Geometry check sheet. Reference: the model listing, model coordinates, mm. A direction names the side the tool comes from. Round coordinates to 2 decimals unless told otherwise and drop trailing zeros. Write each loop counter-clockwise with the first axis right and the second up, starting at its lowest first coordinate (ties: lowest second). Pieces come first, ordered by that corner, then holes. Notation, with made-up numbers: (40, 19) -> (69, 19) arc R8 ccw to (69, 31) -> close; hole circle Ø2 at (22.5, 48). An arc over 180 degrees is marked (long way). One line per question, with ' | ' between items.
```python
from build123d import *

# Parameters (mm, degrees)
ESQUISSE1_R             = 2.5
EXTRUSION1_DEPTH        = 14
ENL_V_MAT_EXTRU_1_DEPTH = 4
ESQUISSE4_R             = 2.5
ENL_V_MAT_EXTRU_2_DEPTH = 3
CHANFREIN1_SIZE         = 1


with BuildPart() as part:
    # Esquisse1 → Extrusion1 (new body)
    with BuildSketch(Plane.XY):
        with BuildLine():
            Line((-1.673913043, 5.239085333), (-12.108695652, 1.905121939))
            ThreePointArc((-12.108695652, 1.905121939), (-13.5, 0), (-12.108695652, -1.905121939))
            Line((-12.108695652, -1.905121939), (-1.673913043, -5.239085333))
            ThreePointArc((-1.673913043, -5.239085333), (5.5, 0), (-1.673913043, 5.239085333))
        make_face()
        Circle(ESQUISSE1_R, mode=Mode.SUBTRACT)
    extrude(amount=EXTRUSION1_DEPTH)

    # Esquisse2 → Enlèv. mat.-Extru.1 (cut)
    with BuildSketch(Plane.XY.offset(14)):
        with BuildLine():
            Line((-1.673913043, 5.239085333), (-7.389278861, 3.412998376))
            Line((-7.389278861, 3.412998376), (-6.298809411, 0))
            Line((-6.298809411, 0), (-7.389278861, -3.412998376))
            Line((-7.389278861, -3.412998376), (-1.673913043, -5.239085333))
            ThreePointArc((-1.673913043, -5.239085333), (5.5, 0), (-1.673913043, 5.239085333))
        make_face()
    extrude(amount=-ENL_V_MAT_EXTRU_1_DEPTH, mode=Mode.SUBTRACT)

    # Esquisse4 → Enlèv. mat.-Extru.2 (cut)
    with BuildSketch(Plane(origin=(0, 0, 0), x_dir=(-1, 0, 0), z_dir=(0, 0, -1))):
        Circle(ESQUISSE4_R)
        with BuildLine():
            Line((1.673913043, -5.239085333), (12.108695652, -1.905121939))
            ThreePointArc((12.108695652, -1.905121939), (13.5, 0), (12.108695652, 1.905121939))
            Line((12.108695652, 1.905121939), (1.673913043, 5.239085333))
            ThreePointArc((1.673913043, 5.239085333), (0.847062769, 5.434379879), (0, 5.5))
            Line((0, 5.5), (-1.881110788, -5.168309414))
            ThreePointArc((-1.881110788, -5.168309414), (-0.10947618, -5.498910344), (1.673913043, -5.239085333))
        make_face()
    extrude(amount=-ENL_V_MAT_EXTRU_2_DEPTH, mode=Mode.SUBTRACT)

    # Chanfrein1
    chanfrein1_edges = [part.edges().sort_by_distance(p)[0] for p in [
        (-2.5, 0, 10),
    ]]
    chamfer(chanfrein1_edges, length=CHANFREIN1_SIZE)


solid = part.part
```
(1) Go/stop test with flat-tipped pins: pin 1 (1.5 mm diameter, centred on x = -3.5, z = 9, fed in from +Y); pin 2 (6.5 mm diameter, centred on x = 0, y = 0, fed in from +Z); pin 3 (4 mm diameter, centred on x = -5, y = -4, fed in from +Z). Record where each tip stops, or that it passes through.
Resolved:
pin 1: stops at y = 4.9 | pin 2: stops at z = 9.75 | pin 3: stops at z = 10
(2) Access from +Z, -Z, +X, -X, +Y, -Y to the whole of each face (thin tool, end or side, straight path). Record for faces 1 (the flat face through (0.266, 3.992, 1.479)), 2 (the flat face through (-6.85, 1.73, 12.03)), 3 (the flat face through (-6.836, -1.683, 12.028)).
Resolved:
face 1: -Z, -X, -Y | face 2: +Z, +X, +Y | face 3: +Z, +X, -Y
(3) Sectioned sample at D-D on x = -8.75. Record the cut outline in (y, z), then the cut area to 3 significant figures.
Resolved:
outline: (-2.98, 3) -> (2.98, 3) -> (2.98, 14) -> (-2.98, 14) -> close | area: 65.5 mm2
(4) Sectioned sample at C-C on x = -11.75. Record the cut outline in (y, z).
Resolved:
outline: (-2.02, 3) -> (2.02, 3) -> (2.02, 14) -> (-2.02, 14) -> close
(5) Material ranges on line 1 (Y direction, x = 0, z = 3.5); line 2 (X direction, y = 0, z = 7); line 3 (Z direction, x = -8.5, y = 2), recorded low to high.
Resolved:
line 1: y = -5.5 to -2.5, 2.5 to 5.5 | line 2: x = -13.5 to -2.5, 2.5 to 5.5 | line 3: z = 3 to 14
(6) Sectioned sample at A-A on z = 4.75. Record the cut outline in (x, y).
Resolved:
outline: (-12.11, -1.91) -> (-1.67, -5.24) arc R5.5 ccw (long way) to (-1.67, 5.24) -> (-12.11, 1.91) arc R2 ccw to start; hole circle Ø5 at (0, 0)
(7) Sectioned sample at B-B on z = 11. Record the cut outline in (x, y), then the cut area to 3 significant figures.
Resolved:
outline: (-12.11, -1.91) -> (-7.39, -3.41) -> (-6.3, 0) -> (-7.39, 3.41) -> (-12.11, 1.91) arc R2 ccw to start | area: 32.7 mm2
